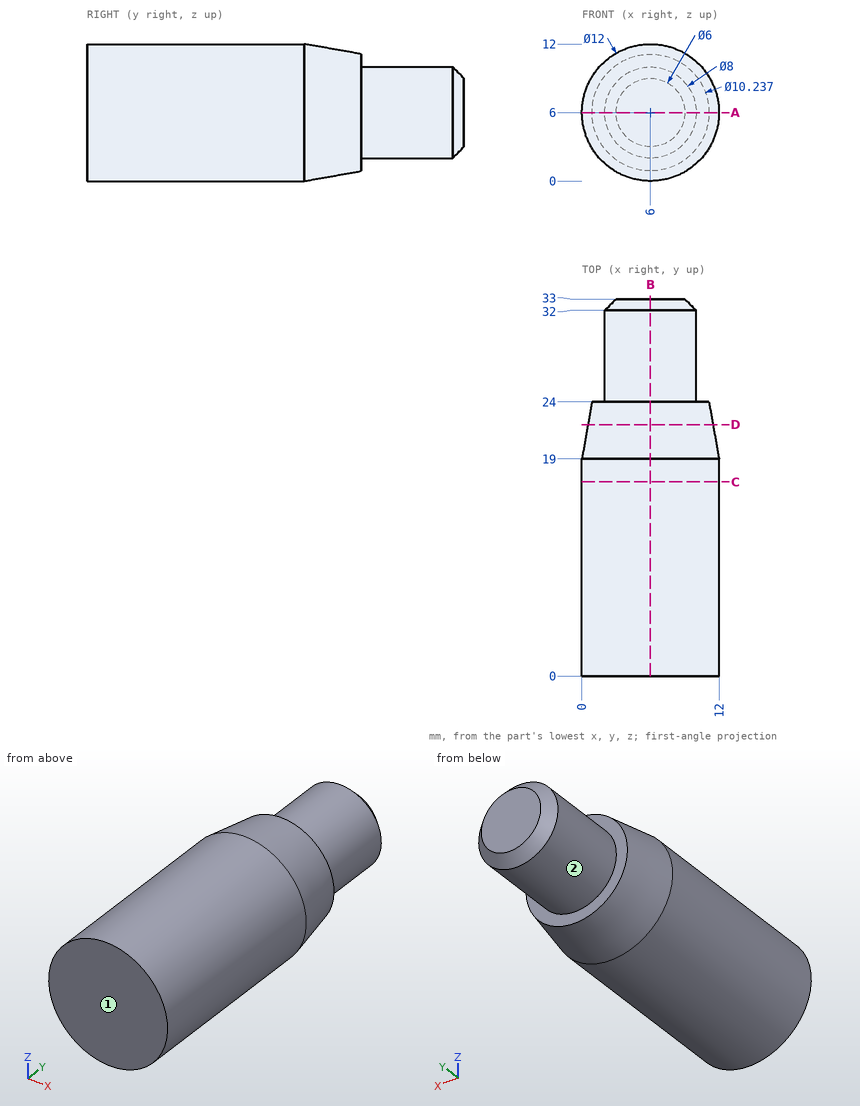
Check sheet for the drawn part. Datum: minimum x, y, z corner. Units: mm. A direction names the side the tool comes from. Coordinates: 2 decimals unless noted, no trailing zeros. Order: outer loops, then holes, each group sorted by start corner. A loop starts at its lowest first (then second) coordinate and runs counter-clockwise, first axis right, second up. Notation, with made-up numbers: (74, 32.25) - (124, 32.25) arc R32 cw to (124, 70.25) - close; hole circle Ø7 at (50.5, 47). An arc over 180 degrees is marked (long way). Return JSON: item names as keys, results as strings.
(1) Go/stop test with flat-tipped pins: pin 1 (6 mm diameter, centred on x = 10.5, y = 29.5, fed in from +Z); pin 2 (4 mm diameter, centred on x = 8.5, y = 9, fed in from +Z). Record where each tip stops, or that it passes through.
Filled sheet:
{"pin 1": "stops at z = 9.71", "pin 2": "stops at z = 11.98"}
(2) Thickness scan on line 1 along X through (y, z) = (12, 5.75) (1 decimal); line 2 along Y through (x, z) = (10, 7.5); line 3 along X through (y, z) = (7, 8.5) (1 decimal). Record the ranges inside material, lowest first.
Filled sheet:
{"line 1": "x = 0 to 12", "line 2": "y = 0 to 24", "line 3": "x = 0.5 to 11.5"}
(3) Access from +Z, -Z, +X, -X, +Y, -Y to the whole of each face (thin tool, end or side, straight path). Record for the marked faces 1 and 2.
Filled sheet:
{"face 1": "+Z, -Z, +X, -X, -Y", "face 2": "+Y"}
(4) Section check A-A, the plane z = 6. Record the cut outline in (x, y).
Filled sheet:
{"outline": "(0, 0) - (12, 0) - (12, 19) - (11.12, 24) - (10, 24) - (10, 32) - (9, 33) - (3, 33) - (2, 32) - (2, 24) - (0.88, 24) - (0, 19) - close"}
(5) Section check D-D, the plane y = 22. Record the cut outline in (x, z).
Filled sheet:
{"outline": "circle Ø10.94 at (6, 6)"}
(6) Section check C-C, the plane y = 17. Record the cut outline in (x, z).
Filled sheet:
{"outline": "circle Ø12 at (6, 6)"}
(7) Section check B-B, the plane x = 6. Record the cut outline in (y, z).
Filled sheet:
{"outline": "(0, 0) - (19, 0) - (24, 0.88) - (24, 2) - (32, 2) - (33, 3) - (33, 9) - (32, 10) - (24, 10) - (24, 11.12) - (19, 12) - (0, 12) - close"}
